```python
from build123d import *

# Parameters (mm, degrees)
SKETCH1_R                  = 5
SKETCH1_R_2                = 2
BOSS_EXTRUDE1_DEPTH        = 3.575
SKETCH2_R                  = 7.5
SKETCH2_R_2                = 2
BOSS_EXTRUDE2_DEPTH        = 1.5
SKETCH3_W                  = 11.269871592
SKETCH3_H                  = 12.441128044
SKETCH3_W_2                = 8.898049958
SKETCH3_H_2                = 8.898049958
CUT_EXTRUDE1_DEPTH         = 7.15
M3X0_5_TAPPED_HOLE1_REACH  = 16.993
M3X0_5_TAPPED_HOLE1_BORE_R = 1.25
SKETCH9_R                  = 3
SKETCH9_R_2                = 2
BOSS_EXTRUDE3_DEPTH        = 7.5
SKETCH11_R                 = 2
BOSS_EXTRUDE4_DEPTH        = 7.5
M3X0_5_TAPPED_HOLE2_D      = 2.5
SKETCH15_R                 = 2
SKETCH15_R_2               = 1.25
CUT_EXTRUDE2_DEPTH         = 2


with BuildPart() as part:
    # Sketch1 → Boss-Extrude1 (new, symmetric)
    with BuildSketch(Plane(origin=(0, 0, 0), x_dir=(1, 0, 0), z_dir=(0, 1, 0))):
        with Locations(Location((0, 0, 0), (0, 0, 270))):
            Circle(SKETCH1_R)
        with Locations(Location((0, 0, 0), (0, 0, 270))):
            Circle(SKETCH1_R_2, mode=Mode.SUBTRACT)
    extrude(amount=BOSS_EXTRUDE1_DEPTH, both=True)

    # Sketch2 → Boss-Extrude2 (add)
    with BuildSketch(Plane(origin=(0, 3.575, 0), x_dir=(1, 0, 0), z_dir=(0, 1, 0))):
        with Locations(Location((0, 0, 0), (0, 0, 270))):
            Circle(SKETCH2_R)
        with Locations(Location((0, 0, 0), (0, 0, 270))):
            Circle(SKETCH2_R_2, mode=Mode.SUBTRACT)
    extrude(amount=BOSS_EXTRUDE2_DEPTH)

    # Sketch3 → Cut-Extrude1 (cut)
    with BuildSketch(Plane.XZ.offset(3.575)):
        Rectangle(SKETCH3_W, SKETCH3_H)
        Rectangle(SKETCH3_W_2, SKETCH3_H_2, mode=Mode.SUBTRACT)
    extrude(amount=-CUT_EXTRUDE1_DEPTH, mode=Mode.SUBTRACT)

    # M3x0.5 Tapped Hole1 bore → M3x0.5 Tapped Hole1 (cut, up to next)
    with BuildSketch(Plane(origin=(0, 0, -4.449024979), x_dir=(-1, 0, 0), z_dir=(0, 0, -1)), mode=Mode.PRIVATE) as m3x0_5_tapped_hole1_sk1:
        with Locations((0, -0.575)):
            Circle(M3X0_5_TAPPED_HOLE1_BORE_R)
    m3x0_5_tapped_hole1_tool1 = extrude(m3x0_5_tapped_hole1_sk1.sketch, amount=-M3X0_5_TAPPED_HOLE1_REACH, mode=Mode.PRIVATE) & part.part
    add(m3x0_5_tapped_hole1_tool1.solids().sort_by_distance((0, -0.575, -4.449025))[0], mode=Mode.SUBTRACT)

    # Sketch9 → Boss-Extrude3 (add)
    with BuildSketch(Plane(origin=(0, 5.075, 0), x_dir=(1, 0, 0), z_dir=(0, 1, 0))):
        with Locations(Location((0, 0, 0), (0, 0, 270))):
            Circle(SKETCH9_R)
        with Locations(Location((0, 0, 0), (0, 0, 270))):
            Circle(SKETCH9_R_2, mode=Mode.SUBTRACT)
    extrude(amount=BOSS_EXTRUDE3_DEPTH)

    # Sketch11 → Boss-Extrude4 (add)
    with BuildSketch(Plane(origin=(0, 12.575, 0), x_dir=(1, 0, 0), z_dir=(0, 1, 0))):
        with Locations(Location((0, 0, 0), (0, 0, 270))):
            Circle(SKETCH11_R)
    extrude(amount=-BOSS_EXTRUDE4_DEPTH)

    # M3x0.5 Tapped Hole2 (through all)
    with Locations(Plane(origin=(0, 12.575, 0), x_dir=(1, 0, 0), z_dir=(0, 1, 0))):
        with Locations((0, 0)):
            Hole(M3X0_5_TAPPED_HOLE2_D / 2)

    # Sketch15 → Cut-Extrude2 (cut)
    with BuildSketch(Plane.XZ.offset(-5.075)):
        with Locations(Location((0, 0, 0), (0, 0, 270))):
            Circle(SKETCH15_R)
        with Locations(Location((0, 0, 0), (0, 0, 90))):
            Circle(SKETCH15_R_2, mode=Mode.SUBTRACT)
    extrude(amount=-CUT_EXTRUDE2_DEPTH, mode=Mode.SUBTRACT)


solid = part.part
```
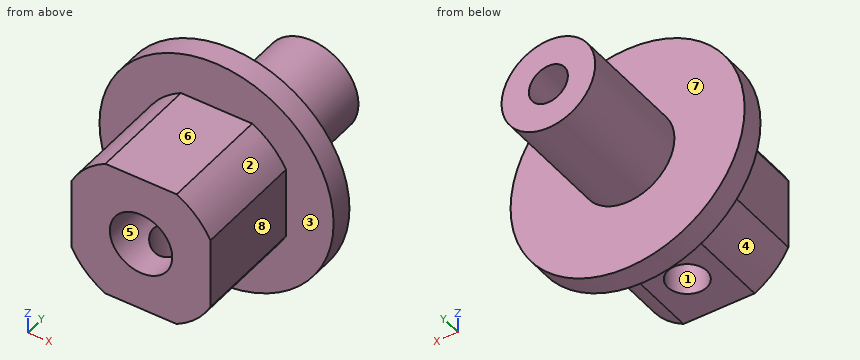
Check sheet for the modelled part. Datum: model origin and axes. Units: mm. Face numbers are marked on the shaded views. A direction names the side the tool comes from. Coordinates: 2 decimals unless noted, no trailing zeros. Loops run counter-clockwise (first coordinate to the right, second up) from the corner with the lowest first, then second, coordinate; pieces in that order, holes last.
1) Sectioned sample at C-C (z = -2.5). Record the boundary of the cut face in (x, y) (3 decimals), and give its area (3 significant figures).
2) Access from +Z, -Z, +X, -X, +Y, -Y to the whole of each face (thin tool, end or side, straight path). Record for the marked faces 4, 5, 6, 7 and 8.
3) Sectioned sample at D-D (y = 4). Record the boundary of the cut face in (x, z), and give its area (3 significant figures).
4) Release check for a two-part mould opening along Y. For the marked faces 1, 2 and 3 record: released by +Y, released by -Y, zero draft, split by the parting line, or undercut.
5) Sectioned sample at A-A (x = 0). Record the boundary of the cut face in (y, z) (3 decimals).
6) Sectioned sample at B-B (z = 0). Record the boundary of the cut face in (x, y) (3 decimals), and give its area (3 significant figures).
7) Material ranges on probe 1 along X at (y, z) = (3.75, 0); probe 2 along Y at (x, z) = (-2.5, -3.25) (3 decimals); probe 3 along Y at (x, z) = (-3, 4.5) (3 decimals), recorded low to high.
8) Gauge pin test, flat ends, axial feed: pin 1 (2 mm diameter, centred on y = 10, z = -1, fed in from +X); pin 2 (1.4 mm diameter, centred on x = -1, y = 1, fed in from +Z); pin 3 (5 mm diameter, centred on y = -0.5, z = 0, fed in from -X); pin 4 (1.5 mm diameter, centred on x = 4, y = 9.5, fed in from -Z). Record the tip position at first contact, or that the pin passes through.
Check sheet entries:
1. outline: (-7.071, 3.575) - (-4.33, 3.575) - (-4.33, -3.575) - (4.33, -3.575) - (4.33, 3.575) - (7.071, 3.575) - (7.071, 5.075) - (1.658, 5.075) - (1.658, 12.575) - (-1.658, 12.575) - (-1.658, 5.075) - (-7.071, 5.075) - close; hole circle Ø2.5 at (0, -0.575)
1. area: 103 mm2
2. face 4: -Z, -X, -Y
2. face 5: -Y
2. face 6: +Z, +X, -X, -Y
2. face 7: +Y
2. face 8: +Z, -Z, +X, -Y
3. outline: circle Ø15 at (0, 0); hole circle Ø4 at (0, 0)
3. area: 164 mm2
4. face 1: undercut
4. face 2: zero draft
4. face 3: released by -Y
5. outline: (-3.575, -4.449) - (-1.825, -4.449) - (-1.825, -2) - (-3.575, -2) - close; (-3.575, 2) - (7.075, 2) - (7.075, 1.25) - (12.575, 1.25) - (12.575, 3) - (5.075, 3) - (5.075, 7.5) - (3.575, 7.5) - (3.575, 4.449) - (-3.575, 4.449) - close; (0.675, -4.449) - (3.575, -4.449) - (3.575, -7.5) - (5.075, -7.5) - (5.075, -3) - (12.575, -3) - (12.575, -1.25) - (7.075, -1.25) - (7.075, -2) - (0.675, -2) - close
6. outline: (-7.5, 3.575) - (-4.449, 3.575) - (-4.449, -3.575) - (-2, -3.575) - (-2, 7.075) - (-1.25, 7.075) - (-1.25, 12.575) - (-3, 12.575) - (-3, 5.075) - (-7.5, 5.075) - close; (1.25, 7.075) - (2, 7.075) - (2, -3.575) - (4.449, -3.575) - (4.449, 3.575) - (7.5, 3.575) - (7.5, 5.075) - (3, 5.075) - (3, 12.575) - (1.25, 12.575) - close
6. area: 74.8 mm2
7. probe 1: x = -7.5 to -2, 2 to 7.5
7. probe 2: y = -3.575 to 5.075
7. probe 3: y = 3.575 to 5.075
8. pin 1: stops at x = 3
8. pin 2: stops at z = 4.45
8. pin 3: stops at x = -4.45
8. pin 4: passes through
